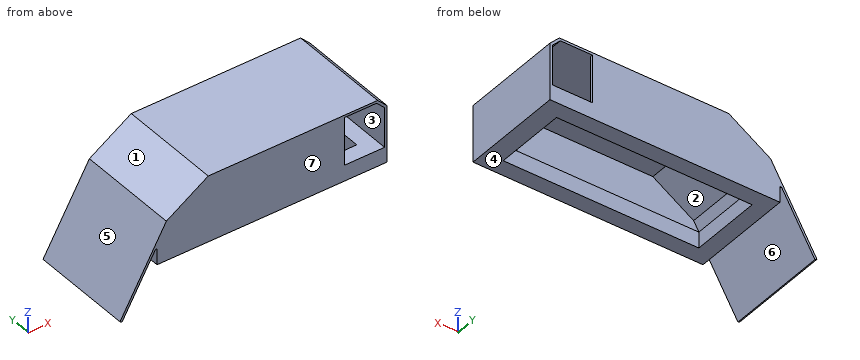
from build123d import *

# Parameters (mm, degrees)
SKETCH1_W           = 285
SKETCH1_H           = 130
SKETCH1_W_2         = 245
SKETCH1_H_2         = 90
BOSS_EXTRUDE1_DEPTH = 20
EXTRUDE_THIN1_DEPTH = 130
BOSS_EXTRUDE2_REACH = 399.778
BOSS_EXTRUDE2_START = 50
SKETCH3_W           = 60
SKETCH3_H           = 3


with BuildPart() as part:
    # Sketch1 → Boss-Extrude1 (new body)
    with BuildSketch(Plane.XY):
        Rectangle(SKETCH1_W, SKETCH1_H)
        Rectangle(SKETCH1_W_2, SKETCH1_H_2, mode=Mode.SUBTRACT)
    extrude(amount=BOSS_EXTRUDE1_DEPTH)

    # Sketch2 → Extrude-Thin1 (add, through all)
    with BuildSketch(Plane(origin=(0, 65, 0), x_dir=(1, 0, 0), z_dir=(0, 1, 0))):
        Polygon((-186.31677691, 52.520571585), (-128.581749991, -47.479428415), (-77.5, -80), (132.5, -80), (142.5, -70), (142.5, 0), (145.5, 0), (145.5, -71.242640687), (133.742640687, -83), (-78.373919532, -83), (-130.812533941, -49.615597272), (-188.914853122, 51.020571585), align=None)
    extrude(amount=-EXTRUDE_THIN1_DEPTH)

    # Sketch3 → Boss-Extrude2 (add, up to next)
    with BuildSketch(Plane.ZY.offset(-142.5).offset(BOSS_EXTRUDE2_START), mode=Mode.PRIVATE) as boss_extrude2_sk1:
        with Locations((50, -63.5)):
            Rectangle(SKETCH3_W, SKETCH3_H)
    boss_extrude2_tool1 = extrude(boss_extrude2_sk1.sketch, amount=BOSS_EXTRUDE2_REACH, mode=Mode.PRIVATE) - part.part
    # Sketch3 → Boss-Extrude2 (add, up to next)
    with BuildSketch(Plane.ZY.offset(-142.5).offset(BOSS_EXTRUDE2_START), mode=Mode.PRIVATE) as boss_extrude2_sk2:
        with Locations((50, 63.5)):
            Rectangle(SKETCH3_W, SKETCH3_H)
    boss_extrude2_tool2 = extrude(boss_extrude2_sk2.sketch, amount=BOSS_EXTRUDE2_REACH, mode=Mode.PRIVATE) - part.part
    add(boss_extrude2_tool1.solids().sort_by_distance((92.5, -63.5, 50))[0])
    add(boss_extrude2_tool2.solids().sort_by_distance((92.5, 63.5, 50))[0])


solid = part.part
Input: part model. Units: mm. Frame: model coordinates. Face numbers are marked on the shaded views. A direction names the side the tool comes from. Give positions to 0.01 mm unless a question says otherwise; leave off trailing zeros. Write each loop counter-clockwise with the first axis right and the second up, starting at its lowest first coordinate (ties: lowest second). Pieces come first, ordered by that corner, then holes.
Q1. Set-up query: the marked faces 1, 2 and 3. Return all of +Z, -Z, +X, -X, +Y, -Y with unobstructed straight access to the full face (end or side cutting, diameter ignored); none if empty.
Q2. Section C-C, the plane z = 8.5. Output: boundary loops of the cut face in (x, y).
Q3. Pull-direction query (Z, two-part tool) for the marked faces 4, 5, 6 and 7; classes: pulls with the +Z half, pulls with the -Z half, needs draft (parallel to the pull), parting line crosses it, or undercut.
Q4. Section B-B, the plane y = 27. Output: boundary loops of the cut face in (x, z).
Q5. Section D-D, the plane z = 60.5. Output: boundary loops of the cut face in (x, y).
Q6. Material intervals for probe 1 along Z at (x, y) = (4.5, 49.5); probe 2 along Y at (x, z) = (-24.5, 61); probe 3 along Y at (x, z) = (-83, 2.5), sorted ascending.
Q7. Section A-A, the plane x = 116.5. Output: boundary loops of the cut face in (y, z), plus the area to 3 significant figures.
Q8. First-contact query: P1, Ø15, axis at y = 6, z = 51, coming from the -X side; P2, Ø3, axis at y = 51.5, z = 34.5, coming from the -X side; P3, Ø1, axis at x = -143.5, y = -64, coming from the -Z side. Flat tips, straight axial feed; report the tip coordinate or a pass-through.
Filled in:
1. face 1: +Z, -X, +Y, -Y
1. face 2: none
1. face 3: +Y, -Y
2. outline: (-154.55, -65) - (-151.09, -65) - (-151.09, 65) - (-154.55, 65) - close; (-142.5, -65) - (145.5, -65) - (145.5, 65) - (-142.5, 65) - close; hole (-122.5, -45) - (122.5, -45) - (122.5, 45) - (-122.5, 45) - close
3. face 4: pulls with the -Z half
3. face 5: pulls with the +Z half
3. face 6: undercut
3. face 7: needs draft
4. outline: (-188.91, -51.02) - (-186.32, -52.52) - (-128.58, 47.48) - (-77.5, 80) - (132.5, 80) - (142.5, 70) - (142.5, 20) - (122.5, 20) - (122.5, 0) - (145.5, 0) - (145.5, 71.24) - (133.74, 83) - (-78.37, 83) - (-130.81, 49.62) - close; (-142.5, 0) - (-122.5, 0) - (-122.5, 20) - (-142.5, 20) - close
5. outline: (-113.72, -65) - (92.5, -65) - (92.5, -62) - (-108.13, -62) - (-108.13, 62) - (92.5, 62) - (92.5, 65) - (-113.72, 65) - close; (142.5, -65) - (145.5, -65) - (145.5, 65) - (142.5, 65) - close
6. probe 1: z = 0 to 20, 80 to 83
6. probe 2: y = -65 to -62, 62 to 65
6. probe 3: y = -65 to -45, 45 to 65
7. outline: (-65, 0) - (-45, 0) - (-45, 20) - (-65, 20) - close; (-65, 80) - (65, 80) - (65, 83) - (-65, 83) - close; (45, 0) - (65, 0) - (65, 20) - (45, 20) - close
7. area: 1,190 mm2
8. P1: stops at x = -134.34
8. P2: stops at x = -140.41
8. P3: stops at z = 20
